```python
from build123d import *

# Parameters (mm, degrees)
SKETCH_1_W          = 70
SKETCH_1_H          = 95
EXTRUDE_1_DEPTH     = 6
SKETCH_2_R          = 4
CUT_EXTRUDE_1_DEPTH = 3.5
SKETCH_3_R          = 1.6
CUT_EXTRUDE_2_DEPTH = 65.065587298
SHELL_1_DEPTH       = 3
FILLET_1_R          = 1.5


# Read off the part's stored shape, not the designer's step: 抽壳1
with BuildPart() as part:
    # 草图1 → 凸台-拉伸1 (new body)
    with BuildSketch(Plane.XY):
        with Locations((1.898047722, -4.528199566)):
            Rectangle(SKETCH_1_W, SKETCH_1_H)
    extrude(amount=EXTRUDE_1_DEPTH)

    # 草图2 → 切除-拉伸1 (cut)
    with BuildSketch(Plane.XY.offset(6)):
        with Locations((30.898047722, 36.971800434)):
            Circle(SKETCH_2_R)
        with Locations((-27.101952278, 36.971800434)):
            Circle(SKETCH_2_R)
        with Locations((30.898047722, -46.028199566)):
            Circle(SKETCH_2_R)
        with Locations((-27.101952278, -46.028199566)):
            Circle(SKETCH_2_R)
    extrude(amount=-CUT_EXTRUDE_1_DEPTH, mode=Mode.SUBTRACT)

    # 草图3 → 切除-拉伸2 (cut, through all)
    with BuildSketch(Plane.XY.offset(6)):
        with Locations((30.898047722, 36.971800434)):
            Circle(SKETCH_3_R)
        with Locations((-27.101952278, 36.971800434)):
            Circle(SKETCH_3_R)
        with Locations((-27.101952278, -46.028199566)):
            Circle(SKETCH_3_R)
        with Locations((30.898047722, -46.028199566)):
            Circle(SKETCH_3_R)
    extrude(amount=-CUT_EXTRUDE_2_DEPTH, mode=Mode.SUBTRACT)

    # 抽壳1 outline → 抽壳1 (cut)
    with BuildSketch(Plane.XY):
        with BuildLine():
            Line((-30.101952278, 30.647245114), (-30.101952278, -39.703644246))
            ThreePointArc((-30.101952278, -39.703644246), (-22.152204809, -41.078452098), (-20.777396957, -49.028199566))
            Line((-20.777396957, -49.028199566), (24.573492402, -49.028199566))
            ThreePointArc((24.573492402, -49.028199566), (25.948300254, -41.078452098), (33.898047722, -39.703644246))
            Line((33.898047722, -39.703644246), (33.898047722, 30.647245114))
            ThreePointArc((33.898047722, 30.647245114), (25.948300254, 32.022052966), (24.573492402, 39.971800434))
            Line((24.573492402, 39.971800434), (-20.777396957, 39.971800434))
            ThreePointArc((-20.777396957, 39.971800434), (-22.152204809, 32.022052966), (-30.101952278, 30.647245114))
        make_face()
    extrude(amount=SHELL_1_DEPTH, mode=Mode.SUBTRACT)

    # 圆角1
    fillet_1_edges = [part.edges().sort_by_distance(p)[0] for p in [
        (36.898047722, -4.528199566, 6),
        (1.898047722, 42.971800434, 6),
        (-33.101952278, -4.528199566, 6),
        (-33.101952278, 42.971800434, 3),
        (36.898047722, 42.971800434, 3),
        (36.898047722, -52.028199566, 3),
        (-33.101952278, -52.028199566, 3),
        (1.898047722, -52.028199566, 6),
    ]]
    fillet(fillet_1_edges, radius=FILLET_1_R)


solid = part.part
```
Source: CAD feature listing. Evaluate the final solid. Frame: model axes, mm. A direction names the side the tool comes from. Give positions to 0.01 mm unless a question says otherwise; leave off trailing zeros. Loops run counter-clockwise (first coordinate to the right, second up) from the corner with the lowest first, then second, coordinate; pieces in that order, holes last. Notation, with made-up numbers: M -28.75,22 L 16.25,22 A26 cw 16.25,40 Z; hole C 10,59 d1. An arc over 180 degrees is marked long. Put each result on its own line as item: value.
Q1. Section A-A (y = -33). Return the cut outline in (x, z), and give its area (3 significant figures).
Response values:
outline: M -33.1,0 L -30.1,0 L -30.1,3 L 33.9,3 L 33.9,0 L 36.9,0 L 36.9,4.5 A1.5 ccw 35.4,6 L -31.6,6 A1.5 ccw -33.1,4.5 Z
area: 227 mm²
Q2. Mould query, pull axis Y, two halves, no side actions, for faces 4 (the flat face through (-30.102, -4, 1)), 5 (the flat face through (36.898, -5, 2)). Classes: released by +Y, released by -Y, zero draft, split by the parting line, or undercut.
Response values:
face 4: undercut
face 5: zero draft
Q3. Section C-C (x = -4). Return the cut outline in (y, z).
Response values:
outline: M -52.03,0 L -49.03,0 L -49.03,3 L 39.97,3 L 39.97,0 L 42.97,0 L 42.97,4.5 A1.5 ccw 41.47,6 L -50.53,6 A1.5 ccw -52.03,4.5 Z
Q4. Section B-B (z = 1.55). Return the cut outline in (x, y).
Response values:
outline: M -33.1,-50.53 A1.5 ccw -31.6,-52.03 L 35.4,-52.03 A1.5 ccw 36.9,-50.53 L 36.9,41.47 A1.5 ccw 35.4,42.97 L -31.6,42.97 A1.5 ccw -33.1,41.47 Z; hole M -30.1,-39.7 A7 cw -20.78,-49.03 L 24.57,-49.03 A7 cw 33.9,-39.7 L 33.9,30.65 A7 cw 24.57,39.97 L -20.78,39.97 A7 cw -30.1,30.65 Z; hole C -27.1,-46.03 d3.2; hole C -27.1,36.97 d3.2; hole C 30.9,-46.03 d3.2; hole C 30.9,36.97 d3.2
Q5. Line query: probe 1 along X at (y, z) = (-8.5, 2.3); probe 2 along X at (y, z) = (-45.5, 3.3); probe 3 along Y at (x, z) = (-9, 0.65). Output: solid intervals per line, ascending. Write a range as [from, to].
Response values:
probe 1: x = [-33.1, -30.1], [33.9, 36.9]
probe 2: x = [-33.1, -31.07], [-23.14, 26.93], [34.86, 36.9]
probe 3: y = [-52.03, -49.03], [39.97, 42.97]
Q6. Pin query (flat end, axial travel): P1, Ø7, axis at x = -27.1, y = 36.97, coming from the +Z side; P2, Ø3, axis at x = 30.9, y = -46.03, coming from the -Z side. Return the tip coordinate at first contact, or that it passes through.
Response values:
P1: stops at z = 2.5
P2: passes through
Q7. Reachability of faces 1 (the flat face through (-25, -46, 2.5)), 2 (the flat face through (-33.102, -5, 2)), 3 (the flat face through (33.898, -5, 1)) from +Z, -Z, +X, -X, +Y, -Y: full face, straight path, thin tool, end or side. Return the list, or none.
Response values:
face 1: +Z
face 2: +Z, -Z, -X, +Y, -Y
face 3: -Z
